Source: CAD feature listing. Evaluate the final solid. Frame: model axes, mm. Face numbers are marked on the shaded views. A direction names the side the tool comes from. Give positions to 0.01 mm unless a question says otherwise; leave off trailing zeros. Loops run counter-clockwise (first coordinate to the right, second up) from the corner with the lowest first, then second, coordinate; pieces in that order, holes last.
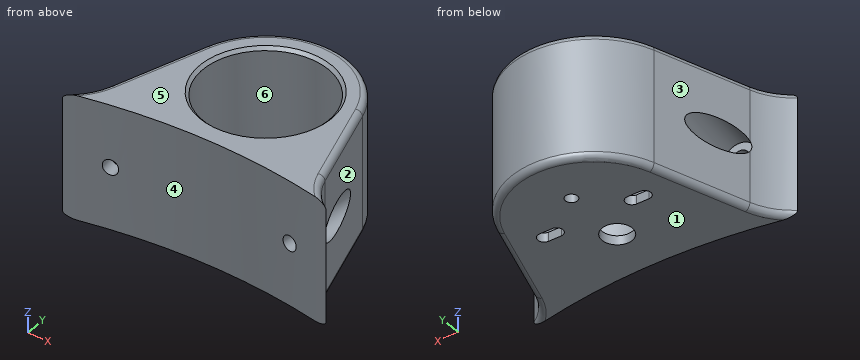
```python
from build123d import *

# Parameters (mm, degrees)
SKETCH1_R           = 26.289
BOSS_EXTRUDE1_DEPTH = 48.26
FILLET1_R           = 2.54
CHAMFER1_SIZE       = 1.27
SKETCH2_R           = 6.35
SKETCH2_R_2         = 2.54
BOSS_EXTRUDE2_DEPTH = 3.81
FILLET2_R           = 2.54
SKETCH4_R           = 3.175
CUT_EXTRUDE1_DEPTH  = 110.759820078
CUT_EXTRUDE2_START  = -6.35
SKETCH5_R           = 6.35
CUT_EXTRUDE2_DEPTH  = 104.409820078


with BuildPart() as part:
    # Sketch1 → Boss-Extrude1 (new body)
    with BuildSketch(Plane.XY):
        with BuildLine():
            Line((-45.642801894, 83.373274477), (-33.240070063, 121.841966324))
            ThreePointArc((-33.240070063, 121.841966324), (0, 146.05), (33.240070063, 121.841966324))
            Line((33.240070063, 121.841966324), (45.642801894, 83.373274477))
            ThreePointArc((45.642801894, 83.373274477), (49.65717276, 75.716693762), (56.007, 69.85))
            ThreePointArc((56.007, 69.85), (0, 76.2), (-56.007, 69.85))
            ThreePointArc((-56.007, 69.85), (-49.65717276, 75.716693762), (-45.642801894, 83.373274477))
        make_face()
        with Locations((0, 111.125)):
            Circle(SKETCH1_R, mode=Mode.SUBTRACT)
    extrude(amount=-BOSS_EXTRUDE1_DEPTH)

    # Fillet1
    fillet1_edges = [part.edges().sort_by_distance(p)[0] for p in [
        (-49.65717276, 75.716693762, 0),
        (-39.441435979, 102.6076204, 0),
        (0, 146.05, 0),
        (39.441435979, 102.6076204, 0),
        (49.65717276, 75.716693762, 0),
    ]]
    fillet(fillet1_edges, radius=FILLET1_R)

    # Chamfer1
    chamfer1_edges = [part.edges().sort_by_distance(p)[0] for p in [
        (-26.289, 111.125, 0),
    ]]
    chamfer(chamfer1_edges, length=CHAMFER1_SIZE)

    # Sketch2 → Boss-Extrude2 (add)
    with BuildSketch(Plane(origin=(0, 0, -48.26), x_dir=(-1, 0, 0), z_dir=(0, 0, -1))):
        with BuildLine():
            Line((45.642801894, 83.373274477), (33.240070063, 121.841966324))
            ThreePointArc((33.240070063, 121.841966324), (0, 146.05), (-33.240070063, 121.841966324))
            Line((-33.240070063, 121.841966324), (-45.642801894, 83.373274477))
            ThreePointArc((-45.642801894, 83.373274477), (-49.65717276, 75.716693762), (-56.007, 69.85))
            ThreePointArc((-56.007, 69.85), (0, 76.2), (56.007, 69.85))
            ThreePointArc((56.007, 69.85), (49.65717276, 75.716693762), (45.642801894, 83.373274477))
        make_face()
        with Locations(Location((0, 97.917, 0), (0, 0, 180))):
            Circle(SKETCH2_R, mode=Mode.SUBTRACT)
        with Locations(Location((0, 124.333, 0), (0, 0, 180))):
            Circle(SKETCH2_R_2, mode=Mode.SUBTRACT)
        with BuildLine():
            Line((-21.336, 113.792), (-16.002, 113.792))
            ThreePointArc((-16.002, 113.792), (-13.335, 111.125), (-16.002, 108.458))
            Line((-16.002, 108.458), (-21.336, 108.458))
            ThreePointArc((-21.336, 108.458), (-24.003, 111.125), (-21.336, 113.792))
        make_face(mode=Mode.SUBTRACT)
        with BuildLine():
            Line((21.336, 113.792), (16.002, 113.792))
            ThreePointArc((16.002, 113.792), (13.335, 111.125), (16.002, 108.458))
            Line((16.002, 108.458), (21.336, 108.458))
            ThreePointArc((21.336, 108.458), (24.003, 111.125), (21.336, 113.792))
        make_face(mode=Mode.SUBTRACT)
    extrude(amount=BOSS_EXTRUDE2_DEPTH)

    # Fillet2
    fillet2_edges = [part.edges().sort_by_distance(p)[0] for p in [
        (-49.65717276, 75.716693762, -52.07),
        (-39.441435979, 102.6076204, -52.07),
        (0, 146.05, -52.07),
        (39.441435979, 102.6076204, -52.07),
        (49.65717276, 75.716693762, -52.07),
    ]]
    fillet(fillet2_edges, radius=FILLET2_R)

    # Sketch4 → Cut-Extrude1 (cut, symmetric)
    with BuildSketch(Plane(origin=(11.899806241, 77.314282605, 0), x_dir=(-0.9883615104677608, 0.15212338618991694, 0), z_dir=(-0.15212338618991694, -0.9883615104677608, 0))):
        with Locations(Location((-26.464277226, 26.035, 0), (0, 0, 180))):
            Circle(SKETCH4_R)
    cut_extrude1 = extrude(amount=CUT_EXTRUDE1_DEPTH, both=True, mode=Mode.SUBTRACT)

    # Sketch5 → Cut-Extrude2 (cut, through all)
    with BuildSketch(Plane(origin=(11.899806241, 77.314282605, 0), x_dir=(-0.9883615104677608, 0.15212338618991694, 0), z_dir=(-0.15212338618991694, -0.9883615104677608, 0)).offset(CUT_EXTRUDE2_START)):
        with Locations(Location((-26.464277226, 26.035, 0), (0, 0, 180))):
            Circle(SKETCH5_R)
    cut_extrude2 = extrude(amount=-CUT_EXTRUDE2_DEPTH, mode=Mode.SUBTRACT)

    # Mirror1: Cut-Extrude1, Cut-Extrude2 across plane
    add(cut_extrude1.mirror(Plane(origin=(0, 0, 0), x_dir=(0, 0, 1), z_dir=(1, 0, 0))), mode=Mode.SUBTRACT)
    add(cut_extrude2.mirror(Plane(origin=(0, 0, 0), x_dir=(0, 0, 1), z_dir=(1, 0, 0))), mode=Mode.SUBTRACT)


solid = part.part
```
(1) Ray query, line 1 along Y through (x, z) = (0, -49.7); line 2 along Y through (x, z) = (0, -27); line 3 along X through (y, z) = (104.5, -21.5). Return the intervals inside material, ascending.
A:
line 1: y = 76.2 to 91.57, 104.27 to 121.79, 126.87 to 146.04
line 2: y = 76.2 to 84.84, 137.41 to 146.05
line 3: x = -38.36 to -25.44, 25.44 to 38.36
(2) Section A-A, the plane x = 0. Return the cut outline in (y, z), then the cut area to 3 significant figures.
A:
outline: (76.2, -52.07) - (91.57, -52.07) - (91.57, -48.26) - (84.84, -48.26) - (84.84, -1.27) - (83.57, 0) - (76.2, 0) - close; (104.27, -52.07) - (121.79, -52.07) - (121.79, -48.26) - (104.27, -48.26) - close; (126.87, -52.07) - (143.51, -52.07) arc R2.54 ccw to (146.05, -49.53) - (146.05, -2.54) arc R2.54 ccw to (143.51, 0) - (138.68, 0) - (137.41, -1.27) - (137.41, -48.26) - (126.87, -48.26) - close
area: 1,030 mm2
(3) Section C-C, the plane z = -6. Return the cut outline in (x, y) (3 decimals).
A:
outline: (-56.007, 69.85) arc R250.166 cw to (56.007, 69.85) arc R25.4 cw to (45.643, 83.373) - (33.24, 121.842) arc R34.925 ccw to (-33.24, 121.842) - (-45.643, 83.373) arc R25.4 cw to start; hole circle Ø52.578 at (0, 111.125)
(4) Mould query, pull axis X, two halves, no side actions, for the marked faces 1, 2, 3 and 4. Classes: pulls with the +X half, pulls with the -X half, needs draft (parallel to the pull), parting line crosses it, or undercut.
A:
face 1: needs draft
face 2: pulls with the +X half
face 3: pulls with the -X half
face 4: undercut
(5) First-contact query: pin 1 (8 mm diameter, centred on y = 102, z = -25, fed in from -X); pin 2 (3 mm diameter, centred on x = -19, z = -51, fed in from +Y); pin 3 (2 mm diameter, centred on x = 29.5, z = -43.5, fed in from +Y). Flat tips, straight axial feed; report the tip coordinate or a pass-through.
A:
pin 1: stops at x = -38.6
pin 2: stops at y = 141.11
pin 3: stops at y = 131.31
(6) Reachability of the marked faces 5 and 6 from +Z, -Z, +X, -X, +Y, -Y: full face, straight path, thin tool, end or side. Return the list, or none.
A:
face 5: +Z, +X, -X, +Y, -Y
face 6: +Z
